Geometry: final body of the model. Coordinates: model frame, mm. Give positions to 0.01 mm unless a question says otherwise; leave off trailing zeros. Write each loop counter-clockwise with the first axis right and the second up, starting at its lowest first coordinate (ties: lowest second). Pieces come first, ordered by that corner, then holes.
Q1. Line query: line 1 (Z direction, x = 7.5, y = 17.75). Output: solid intervals per line, ascending.
Q2. Pin query (flat end, axial travel): pin 1 Ø0.5 at (x, y) = (27.5, 9.5) entering from -Z; pin 2 Ø0.8 at (x, y) = (29.5, 12) entering from +Z. Return the tip coordinate at first contact, or that it passes through.
Q3. Section A-A (x = 17.5). Return the cut outline in (y, z), plus the area to 3 significant figures.
Q4. Section B-B (z = 4.25). State how many separate pieces and enclosed holes the cut face has, plus the area to 3 significant figures.
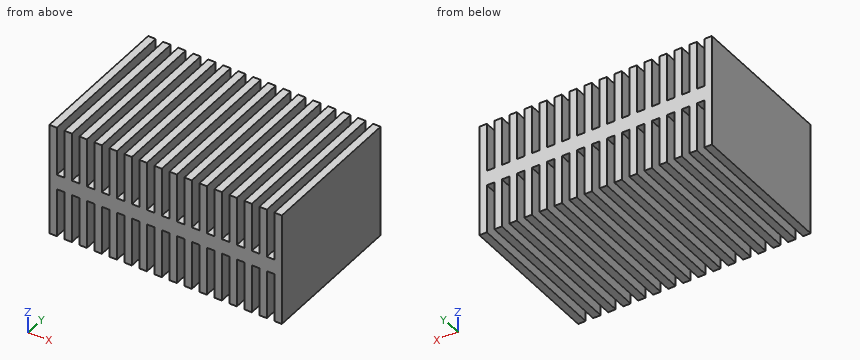
from build123d import *

# Parameters (mm, degrees)
SKETCH2_W           = 1
SKETCH2_H           = 2
BOSS_EXTRUDE1_DEPTH = 20


with BuildPart() as part:
    # Sketch2 → Boss-Extrude1 (new body)
    with BuildSketch(Plane(origin=(0, 0, 0), x_dir=(1, 0, 0), z_dir=(0, 1, 0))):
        Polygon((1, 0), (0, 0), (0, -15), (1, -15), (1, -8.5), (2, -8.5), (2, -6.5), (1, -6.5), align=None)
        Polygon((2, 0), (2, -6.5), (2, -8.5), (2, -15), (3, -15), (3, -8.5), (4, -8.5), (4, -6.5), (3, -6.5), (3, 0), align=None)
        Polygon((4, 0), (4, -6.5), (4, -8.5), (4, -15), (5, -15), (5, -8.5), (6, -8.5), (6, -6.5), (5, -6.5), (5, 0), align=None)
        Polygon((6, 0), (6, -6.5), (6, -8.5), (6, -15), (7, -15), (7, -8.5), (8, -8.5), (8, -6.5), (7, -6.5), (7, 0), align=None)
        Polygon((8, 0), (8, -6.5), (8, -8.5), (8, -15), (9, -15), (9, -8.5), (10, -8.5), (10, -6.5), (9, -6.5), (9, 0), align=None)
        Polygon((10, 0), (10, -6.5), (10, -8.5), (10, -15), (11, -15), (11, -8.5), (12, -8.5), (12, -6.5), (11, -6.5), (11, 0), align=None)
        Polygon((12, 0), (12, -6.5), (12, -8.5), (12, -15), (13, -15), (13, -8.5), (13, -6.5), (13, 0), align=None)
        with Locations((13.5, -7.5)):
            Rectangle(SKETCH2_W, SKETCH2_H)
        Polygon((14, 0), (14, -6.5), (14, -8.5), (14, -15), (15, -15), (15, -8.5), (16, -8.5), (16, -6.5), (15, -6.5), (15, 0), align=None)
        Polygon((16, 0), (16, -6.5), (16, -8.5), (16, -15), (17, -15), (17, -8.5), (18, -8.5), (18, -6.5), (17, -6.5), (17, 0), align=None)
        Polygon((18, 0), (18, -6.5), (18, -8.5), (18, -15), (19, -15), (19, -8.5), (20, -8.5), (20, -6.5), (19, -6.5), (19, 0), align=None)
        Polygon((20, 0), (20, -6.5), (20, -8.5), (20, -15), (21, -15), (21, -8.5), (22, -8.5), (22, -6.5), (21, -6.5), (21, 0), align=None)
        Polygon((22, 0), (22, -6.5), (22, -8.5), (22, -15), (23, -15), (23, -8.5), (24, -8.5), (24, -6.5), (23, -6.5), (23, 0), align=None)
        Polygon((24, 0), (24, -6.5), (24, -8.5), (24, -15), (25, -15), (25, -8.5), (26, -8.5), (26, -6.5), (25, -6.5), (25, 0), align=None)
        Polygon((26, 0), (26, -6.5), (26, -8.5), (26, -15), (27, -15), (27, -8.5), (28, -8.5), (28, -6.5), (27, -6.5), (27, 0), align=None)
        Polygon((28, 0), (28, -6.5), (28, -8.5), (28, -15), (29, -15), (29, -8.5), (30, -8.5), (30, -6.5), (29, -6.5), (29, 0), align=None)
        Polygon((30, 0), (30, -6.5), (30, -8.5), (30, -15), (31, -15), (31, 0), align=None)
    extrude(amount=BOSS_EXTRUDE1_DEPTH)


solid = part.part
Computed:
1. line 1: z = 6.5 to 8.5
2. pin 1: stops at z = 6.5
2. pin 2: stops at z = 8.5
3. outline: (0, 6.5) - (20, 6.5) - (20, 8.5) - (0, 8.5) - close
3. area: 40.0 mm2
4. separate pieces: 16
4. enclosed holes: 0
4. area: 320 mm2
